Part model, mm, in its own coordinate system. A direction names the side the tool comes from. Round coordinates to 2 decimals unless told otherwise and drop trailing zeros. Write each loop counter-clockwise with the first axis right and the second up, starting at its lowest first coordinate (ties: lowest second). Pieces come first, ordered by that corner, then holes. Notation, with made-up numbers: M 28,-23.5 L 82,-23.5 A18 cw 82,3.5 Z; hole C 60,2 d4. An arc over 180 degrees is marked long. Use one line per item in the form item = value. Start each with the question number.
Item 1: Cut at A-A, the plane x = 0. Give the cut face in (y, z).
Item 2: Cut at D-D, the plane x = -17. Give the cut face in (y, z).
Item 3: Which spindle directions (+Z, -Z, +X, -X, +Y, -Y) get a long thin tool onto all of the face, cutting with end or side? Do faces 1 (the face through (-5, 20, 0)), 2 (the face through (-3.905, 14.93, 0.867)), 3 (the face through (5, 10, 0)). Say none if no direction does.
Item 4: Probe L1, parallel to X at y = 25.25, z = 0; L2, parallel to X at y = 14.5, z = 0; L3, parallel to Y at x = -1.5, z = 6.5. List the from-to ranges inside material, lowest first.
Item 5: Mould opens along Z. For faces 4 (the face through (-8.618, 25.07, 20.784)), 5 (the face through (-21, 15, -28)), 6 (the face through (-23, 30, 0)) say: +Z half, -Z half, draft (parallel to the pull), parting line (faces both ways), or undercut.
Item 6: Flat gauge pins, fed straight in: pin 1 Ø6 at (y, z) = (25, -24) entering from +X; pin 2 Ø12 at (x, y) = (14.5, 19.5) entering from +Z; pin 3 Ø1 at (x, z) = (1.5, -17.5) entering from +Y; pin 4 Ø10 at (x, z) = (-12, -13.5) entering from -Y. Where does each tip first touch, or does it go through?
Item 7: Cut at C-C, the plane y = 26.5. Give the cut face in (x, z).
Item 8: Cut at B-B, the plane z = 0. Give the cut face in (x, y).
from build123d import *

# Parameters (mm, degrees)
SKETCH1_R           = 35
BOSS_EXTRUDE1_DEPTH = 30
SKETCH2_R           = 22.5
CUT_EXTRUDE1_DEPTH  = 10
CUT_EXTRUDE2_START  = -10
SKETCH3_R           = 22.5
CUT_EXTRUDE2_DEPTH  = 10
SKETCH4_R           = 4
CUT_EXTRUDE3_DEPTH  = 10


with BuildPart() as part:
    # Sketch1 → Boss-Extrude1 (new body)
    with BuildSketch(Plane(origin=(0, 0, 0), x_dir=(1, 0, 0), z_dir=(0, 1, 0))):
        with Locations(Location((0, 0, 0), (0, 0, 270))):
            Circle(SKETCH1_R)
    extrude(amount=BOSS_EXTRUDE1_DEPTH)

    # Sketch2 → Cut-Extrude1 (cut)
    with BuildSketch(Plane(origin=(0, 30, 0), x_dir=(1, 0, 0), z_dir=(0, 1, 0))):
        with Locations(Location((0, 0, 0), (0, 0, 270))):
            Circle(SKETCH2_R)
    extrude(amount=-CUT_EXTRUDE1_DEPTH, mode=Mode.SUBTRACT)

    # Sketch3 → Cut-Extrude2 (cut)
    with BuildSketch(Plane.XZ.offset(CUT_EXTRUDE2_START)):
        with Locations(Location((0, 0, 0), (0, 0, 90))):
            Circle(SKETCH3_R)
    extrude(amount=CUT_EXTRUDE2_DEPTH, mode=Mode.SUBTRACT)

    # Sketch4 → Cut-Extrude3 (cut)
    with BuildSketch(Plane.XZ.offset(-10)):
        with Locations(Location((0, 0, 0), (0, 0, 270))):
            Circle(SKETCH4_R)
    extrude(amount=-CUT_EXTRUDE3_DEPTH, mode=Mode.SUBTRACT)


solid = part.part
Model answer:
q1.outline = M 0,-35 L 30,-35 L 30,-22.5 L 20,-22.5 L 20,-4 L 10,-4 L 10,-22.5 L 0,-22.5 Z; M 0,22.5 L 10,22.5 L 10,4 L 20,4 L 20,22.5 L 30,22.5 L 30,35 L 0,35 Z
q2.outline = M 0,-30.59 L 30,-30.59 L 30,-14.74 L 20,-14.74 L 20,14.74 L 30,14.74 L 30,30.59 L 0,30.59 L 0,14.74 L 10,14.74 L 10,-14.74 L 0,-14.74 Z
q3.face_1 = +Y
q3.face_2 = +Y, -Y
q3.face_3 = -Y
q4.L1 = -35 to -22.5, 22.5 to 35
q4.L2 = -35 to -4, 4 to 35
q4.L3 = 10 to 20
q5.face_4 = undercut
q5.face_5 = parting line
q5.face_6 = draft
q6.pin_1 = 28
q6.pin_2 = 33.95
q6.pin_3 = 20
q6.pin_4 = 0
q7.outline = C 0,0 d70; hole C 0,0 d45
q8.outline = M -35,0 L -22.5,0 L -22.5,10 L -4,10 L -4,20 L -22.5,20 L -22.5,30 L -35,30 Z; M 4,10 L 22.5,10 L 22.5,0 L 35,0 L 35,30 L 22.5,30 L 22.5,20 L 4,20 Z
